from build123d import *

# Parameters (mm, degrees)
SKETCH4_R                         = 14.2875
CUT_EXTRUDE1_DEPTH                = 407.60558878
CIRPATTERN2_COUNT                 = 28
CIRPATTERN3_COUNT                 = 12
CIRPATTERN4_COUNT                 = 4
CIRPATTERN5_COUNT                 = 4
F_1_2_13_TAPPED_HOLE4_D           = 10.71626
F_1_2_13_TAPPED_HOLE4_DEPTH       = 35.052
F_1_2_13_TAPPED_HOLE4_CSINK_D     = 13.97
F_1_2_13_TAPPED_HOLE4_CSINK_ANGLE = 100
F_1_2_13_TAPPED_HOLE4_TIP         = 3.219489309


with BuildPart() as part:
    # Sketch1 → Revolve1 (revolve)
    with BuildSketch(Plane.XY, mode=Mode.PRIVATE) as revolve1_sk:
        Polygon((-5.9944, 67.7545), (-5.9944, 180.9496), (0, 180.9496), (0, 228.9937), (-5.9944, 228.9937), (-5.9944, 281.051), (28.7528, 281.051), (28.7528, 231.3686), (44.8056, 231.3686), (44.8056, 217.9066), (79.7306, 217.9066), (79.7306, 58.5851), (55.9308, 32.5628), (46.4058, 32.5628), (46.4058, 67.7545), align=None)
    revolve(revolve1_sk.sketch.rotate(Axis((0, 0, 0), (1, 0, 0)), 90), axis=Axis((0, 0, 0), (1, 0, 0)))

    # Sketch4 → Cut-Extrude1 (cut, through all)
    with BuildSketch(Plane.ZY.offset(5.9944)):
        with Locations((28.972111579, 257.135466548)):
            Circle(SKETCH4_R)
    cut_extrude1 = extrude(amount=-CUT_EXTRUDE1_DEPTH, mode=Mode.SUBTRACT)

    # CirPattern2: Cut-Extrude1 ×28 about axis
    cirpattern2_axis = Axis((0, 0, 0), (1, 0, 0))
    for i in range(1, CIRPATTERN2_COUNT):
        add(cut_extrude1.rotate(cirpattern2_axis, i * 360 / CIRPATTERN2_COUNT), mode=Mode.SUBTRACT)

    # Sketch8 → 3/4-10 Tapped Hole1 (revolve, cut)
    with BuildSketch(Plane(origin=(0, 199.3429424, 53.413780433), x_dir=(0, 0, 1), z_dir=(0, 1, 0))):
        Polygon((0, 0), (0, 30.407416175), (8.33374, 25.4), (8.33374, 1.82626), (10.16, 0), align=None)
    f_3_4_10_tapped_hole1 = revolve(axis=Axis((-6.35, 199.3429424, 53.413780433), (1, 0, 0)), mode=Mode.SUBTRACT)

    # CirPattern3: 3/4-10 Tapped Hole1 ×12 about axis
    cirpattern3_axis = Axis((0, 0, 0), (1, 0, 0))
    for i in range(1, CIRPATTERN3_COUNT):
        add(f_3_4_10_tapped_hole1.rotate(cirpattern3_axis, i * 360 / CIRPATTERN3_COUNT), mode=Mode.SUBTRACT)

    # Sketch10 → 7/8-9 Tapped Hole1 (revolve, cut)
    with BuildSketch(Plane(origin=(-5.9944, 67.172315786, 67.172315786), x_dir=(0, 0, 1), z_dir=(0, 1, 0))):
        Polygon((0, 0), (0, 31.242239902), (9.72312, 25.4), (9.72312, 2.02438), (11.7475, 0), align=None)
    f_7_8_9_tapped_hole1 = revolve(axis=Axis((-12.3444, 67.172315786, 67.172315786), (1, 0, 0)), mode=Mode.SUBTRACT)

    # CirPattern4: 7/8-9 Tapped Hole1 ×4 about axis
    cirpattern4_axis = Axis((0, 0, 0), (1, 0, 0))
    for i in range(1, CIRPATTERN4_COUNT):
        add(f_7_8_9_tapped_hole1.rotate(cirpattern4_axis, i * 360 / CIRPATTERN4_COUNT), mode=Mode.SUBTRACT)

    # Sketch12 → Tap Drill for 3/8-16 Tap1 (revolve, cut)
    with BuildSketch(Plane(origin=(-5.9944, -162.844517689, 201.096231852), x_dir=(0, 0, 1), z_dir=(0, 1, 0))):
        Polygon((0, 0), (0, 43.024665582), (3.96875, 40.64), (3.96875, 0.635), (4.60375, 0), align=None)
    tap_drill_for_3_8_16_tap1 = revolve(axis=Axis((-12.3444, -162.844517689, 201.096231852), (1, 0, 0)), mode=Mode.SUBTRACT)

    # CirPattern5: Tap Drill for 3/8-16 Tap1 ×4 about axis
    cirpattern5_axis = Axis((0, 0, 0), (1, 0, 0))
    for i in range(1, CIRPATTERN5_COUNT):
        add(tap_drill_for_3_8_16_tap1.rotate(cirpattern5_axis, i * 360 / CIRPATTERN5_COUNT), mode=Mode.SUBTRACT)

    # 1/2-13 Tapped Hole4
    with Locations(Plane(origin=(11.3792, 281.051, 0), x_dir=(0, 0, 1), z_dir=(0, 1, 0))):
        with Locations((0, 0)):
            CounterSinkHole(F_1_2_13_TAPPED_HOLE4_D / 2, F_1_2_13_TAPPED_HOLE4_CSINK_D / 2, depth=F_1_2_13_TAPPED_HOLE4_DEPTH, counter_sink_angle=F_1_2_13_TAPPED_HOLE4_CSINK_ANGLE)
            with Locations((0, 0, -(F_1_2_13_TAPPED_HOLE4_DEPTH + F_1_2_13_TAPPED_HOLE4_TIP / 2))):  # 118° drill point
                Cone(0, F_1_2_13_TAPPED_HOLE4_D / 2, F_1_2_13_TAPPED_HOLE4_TIP, mode=Mode.SUBTRACT)


solid = part.part
Build history of the part. All positions in model axes, mm. A direction names the side the tool comes from. Give positions to 0.01 mm unless a question says otherwise; leave off trailing zeros. Loops run counter-clockwise (first coordinate to the right, second up) from the corner with the lowest first, then second, coordinate; pieces in that order, holes last. Notation, with made-up numbers: (82, 7.25) - (99, 7.25) arc R17 ccw to (99, 27.25) - close; hole circle Ø10 at (13.5, -8.75). An arc over 180 degrees is marked (long way). Write item = value, one per line. Start each with the question number.
1) Tool access for faces 1 (the cylindrical face through (11.136, 213.301, -124.613)), 2 (the flat face through (46.406, -16, -29)): list every direction of +Z, -Z, +X, -X, +Y, -Y with a clear straight run to the whole face (end or side of a thin tool).
2) Drop flat-ended pins along their axis: pin 1 Ø10 at (x, z) = (18.5, -218.5) entering from -Y; pin 2 Ø1.5 at (x, z) = (17.5, 162) entering from +Y; pin 3 Ø10 at (x, y) = (48, 140.5) entering from +Z. Give the stop position or say it passes through.
3) Probe probe 1 along Z at (x, y) = (22.5, 137); probe 2 along Y at (x, z) = (1.5, 218); probe 3 along Y at (x, z) = (28, -86). List the from-to ranges inside material, lowest first. Write a range as from..to.
4) Band-saw the part on B-B on y = 91. Give the cut face in (x, z).
Final values:
q1.face_1 = +X, -X
q1.face_2 = -X
q2.pin_1 = -182.78
q2.pin_2 = 230.19
q2.pin_3 = 186.7
q3.probe_1 = -245.4..-233.37, -204.83..204.83, 233.37..245.4
q3.probe_2 = -177.39..-151.91, -123.42..123.42, 151.92..177.39
q3.probe_3 = -267.57..-258.52, -229.96..229.96, 258.52..267.57
q4.outline = (-5.99, -265.91) - (28.75, -265.91) - (28.75, -257.41) - (-5.99, -257.41) - close; (-5.99, -231.07) - (28.75, -231.07) - (28.75, -212.72) - (44.81, -212.72) - (44.81, -198) - (79.73, -198) - (79.73, 198) - (44.81, 198) - (44.81, 212.72) - (28.75, 212.72) - (28.75, 231.07) - (-5.99, 231.07) - (-5.99, 210.14) - (0, 210.14) - (0, 156.4) - (-5.99, 156.4) - (-5.99, -156.4) - (0, -156.4) - (0, -210.14) - (-5.99, -210.14) - close; (-5.99, 257.41) - (28.75, 257.41) - (28.75, 265.91) - (-5.99, 265.91) - close
